from build123d import *

# Parameters (mm, degrees)
F0_W     = 1.6
F0_H     = 100
F1_DEPTH = 1.6
F3_DEPTH = 5


with BuildPart() as f1:
    # F0 (on Top) → F1 (new body)
    with BuildSketch(Plane.XY):
        Rectangle(F0_W, F0_H)
    extrude(amount=F1_DEPTH)

    # F2 (on face) → F3 (join)
    with BuildSketch(Plane.XZ.offset(50)):
        with BuildLine():
            Line((-1.111348, 14.30277), (-1.389185, 15.878462))
            ThreePointArc((-1.389185, 15.878462), (-7.99447, 7.702607), (-0.8, 0.040101))
            Line((-0.8, 0.040101), (-0.8, 1.6))
            Line((-0.8, 1.6), (0, 1.6))
            ThreePointArc((0, 1.6), (-6.375646, 7.442203), (-1.111348, 14.30277))
        make_face()
        with BuildLine():
            ThreePointArc((0.8, 0.040101), (5.932959, 2.633437), (8, 8))
            ThreePointArc((8, 8), (6.128356, 13.142301), (1.389185, 15.878462))
            Line((1.389185, 15.878462), (1.111348, 14.30277))
            ThreePointArc((1.111348, 14.30277), (4.902684, 12.113841), (6.4, 8))
            ThreePointArc((6.4, 8), (4.525483, 3.474517), (0, 1.6))
            Line((0, 1.6), (0.8, 1.6))
            Line((0.8, 1.6), (0.8, 0.040101))
        make_face()
        with BuildLine():
            ThreePointArc((0, 0), (0.400502, 0.010031), (0.8, 0.040101))
            Line((0.8, 0.040101), (0.8, 1.6))
            Line((0.8, 1.6), (0, 1.6))
            Line((0, 1.6), (-0.8, 1.6))
            Line((-0.8, 1.6), (-0.8, 0.040101))
            ThreePointArc((-0.8, 0.040101), (-0.400502, 0.010031), (0, 0))
        make_face()
    extrude(amount=F3_DEPTH)


solid = f1.part
Build history of the part. All positions in model axes, mm. Give positions to 0.01 mm unless a question says otherwise; leave off trailing zeros. Loops run counter-clockwise (first coordinate to the right, second up) from the corner with the lowest first, then second, coordinate; pieces in that order, holes last. Notation, with made-up numbers: (67, -19) -> (84, -19) arc R22 ccw to (84, -2) -> close; hole circle Ø5 at (-9.5, 70). An arc over 180 degrees is marked (long way). Answer in a Markdown table with one row per item.
Item 1: Slice it at B-B on x = 5. Write the cut outline in (y, z) (3 decimals).
Findings below:
| item | result |
|---|---|
| outline | (-55, 1.755) -> (-50, 1.755) -> (-50, 4.005) -> (-55, 4.005) -> close; (-55, 11.995) -> (-50, 11.995) -> (-50, 14.245) -> (-55, 14.245) -> close |
Item 2: Probe line 1 along Y through (x, z) = (-6, 10.75). List the from-to ranges inside material, lowest first. Write a range as [from, to].
Findings below:
| item | result |
|---|---|
| line 1 | y = [-55, -50] |
Item 3: Slice it at C-C on y = 16.5. Write the cut outline in (x, z).
Findings below:
| item | result |
|---|---|
| outline | (-0.8, 0) -> (0.8, 0) -> (0.8, 1.6) -> (-0.8, 1.6) -> close |
Item 4: Slice it at A-A on z = 11.5. Write the cut outline in (x, y).
Findings below:
| item | result |
|---|---|
| outline | (-7.19, -55) -> (-5.36, -55) -> (-5.36, -50) -> (-7.19, -50) -> close; (5.36, -55) -> (7.19, -55) -> (7.19, -50) -> (5.36, -50) -> close |
Item 5: Flat gauge pins, fed straight in: P1, Ø2, axis at y = 27.5, z = 4.5, coming from the -X side; P2, Ø6.5, axis at x = -6, z = 10.5, coming from the +Y side; P3, Ø1.8, axis at x = 0, y = -19, coming from the +Z side; P4, Ø0.5, axis at y = 23.5, z = 1, coming from the +X side. Where does each tip first touch, or does it go through?
Findings below:
| item | result |
|---|---|
| P1 | passes through |
| P2 | stops at y = -50 |
| P3 | stops at z = 1.6 |
| P4 | stops at x = 0.8 |
